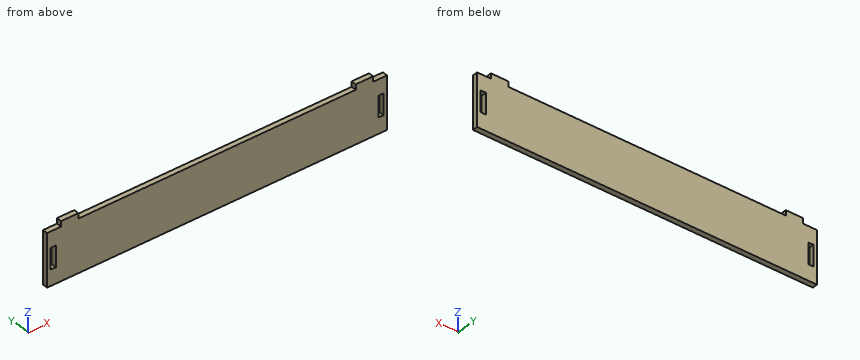
from build123d import *

# Parameters (mm, degrees)
SKETCH_1_W      = 3
SKETCH_1_H      = 12
EXTRUDE_1_DEPTH = 3


with BuildPart() as part:
    # 草图1 → 凸台-拉伸1 (new body)
    with BuildSketch(Plane(origin=(0, 0, 0), x_dir=(1, 0, 0), z_dir=(0, 1, 0))):
        Polygon((-8, 30), (-8, 0), (-3, 0), (0, 0), (0, -3), (10, -3), (10, 0), (170, 0), (170, -3), (180, -3), (180, 0), (183, 0), (188, 0), (188, 30), (183, 30), (180, 30), (0, 30), (-3, 30), align=None)
        with Locations((184.5, 15)):
            Rectangle(SKETCH_1_W, SKETCH_1_H, mode=Mode.SUBTRACT)
        with Locations((-4.5, 15)):
            Rectangle(SKETCH_1_W, SKETCH_1_H, mode=Mode.SUBTRACT)
    extrude(amount=EXTRUDE_1_DEPTH)


solid = part.part
Design review of the part built by this model. Coordinates are the model's own, in mm. Give positions to 0.01 mm unless a question says otherwise; leave off trailing zeros. Loops run counter-clockwise (first coordinate to the right, second up) from the corner with the lowest first, then second, coordinate; pieces in that order, holes last. Notation, with made-up numbers: M 43,82.25 L 95,82.25 A22 ccw 95,109.25 Z; hole C -38,-18 d9. An arc over 180 degrees is marked long. Write item = value, one per line.
Q1. To check wall thickness, follow line 1 (X direction, y = 1.95, z = -15); line 2 (X direction, y = 1.2, z = 0.5); line 3 (Z direction, x = 137, y = 2.45). State the ranges of each line that lie inside material, in increasing order. Write a range as [from, to].
Output values:
line_1 = [-8, -6], [-3, 183], [186, 188]
line_2 = [0, 10], [170, 180]
line_3 = [-30, 0]
Q2. We need section A-A (z = -13). Give the boundary of the cut face in (x, y).
Output values:
outline = M -8,0 L -6,0 L -6,3 L -8,3 Z; M -3,0 L 183,0 L 183,3 L -3,3 Z; M 186,0 L 188,0 L 188,3 L 186,3 Z
Q3. We need section C-C (x = 167). Give the boundary of the cut face in (y, z), plus the area to 3 significant figures.
Output values:
outline = M 0,-30 L 3,-30 L 3,0 L 0,0 Z
area = 90.0 mm^2
Q4. We need section B-B (y = 1). Give the boundary of the cut face in (x, z), plus the area to 3 significant figures.
Output values:
outline = M -8,-30 L 188,-30 L 188,0 L 180,0 L 180,3 L 170,3 L 170,0 L 10,0 L 10,3 L 0,3 L 0,0 L -8,0 Z; hole M -6,-21 L -3,-21 L -3,-9 L -6,-9 Z; hole M 183,-21 L 186,-21 L 186,-9 L 183,-9 Z
area = 5,870 mm^2
Q5. Insertion check: pin 1 (1.5 mm diameter, centred on x = -4.5, y = 1, fed in from +Z); pin 2 (1.5 mm diameter, centred on y = 1, z = 1.5, fed in from -X). Each pin has a flat end and moves straight along its axis. Give the tip position at first contact, or say it passes through.
Output values:
pin_1 = 0
pin_2 = 0
